Could you check a few things on this model? Use its own coordinates, in mm. A direction names the side the tool comes from. Give positions to 0.01 mm unless a question says otherwise; leave off trailing zeros. Loops run counter-clockwise (first coordinate to the right, second up) from the corner with the lowest first, then second, coordinate; pieces in that order, holes last. Notation, with made-up numbers: (29, 47) - (57, 47) arc R10 cw to (57, 57) - close; hole circle Ø8 at (-4, 60.25). An arc over 180 degrees is marked (long way). Write each question's results on one line, items separated by ' | '. Start each with the question number.
```python
from build123d import *

# Parameters (mm, degrees)
EXTRUDE_1_DEPTH     = 12
SKETCH_3_W          = 26
SKETCH_3_H          = 12
CUT_EXTRUDE_1_DEPTH = 2
SKETCH_4_R          = 1.5
CUT_EXTRUDE_2_DEPTH = 7


with BuildPart() as part:
    # 草图2 → 凸台-拉伸1 (new body)
    with BuildSketch(Plane(origin=(0, 0, 0), x_dir=(1, 0, 0), z_dir=(0, 1, 0))):
        Polygon((-13, 0), (-9.07179677, 0), (-8, 4), (8, 4), (9.07179677, 0), (13, 0), (13, 9), (-13, 9), align=None)
    extrude(amount=EXTRUDE_1_DEPTH)

    # 草图3 → 切除-拉伸1 (cut)
    with BuildSketch(Plane(origin=(0, 0, -9), x_dir=(-1, 0, 0), z_dir=(0, 0, -1))):
        with Locations((0, 6)):
            Rectangle(SKETCH_3_W, SKETCH_3_H)
    extrude(amount=-CUT_EXTRUDE_1_DEPTH, mode=Mode.SUBTRACT)

    # 草图4 → 切除-拉伸2 (cut)
    with BuildSketch(Plane(origin=(0, 0, -7), x_dir=(-1, 0, 0), z_dir=(0, 0, -1))):
        with Locations((-11, 3)):
            Circle(SKETCH_4_R)
        with Locations(Location((11, 3, 0), (0, 0, 180))):
            Circle(SKETCH_4_R)
        with Locations((11, 9)):
            Circle(SKETCH_4_R)
        with Locations(Location((-11, 9, 0), (0, 0, 180))):
            Circle(SKETCH_4_R)
    extrude(amount=-CUT_EXTRUDE_2_DEPTH, mode=Mode.SUBTRACT)


solid = part.part
```
Q1. If we mould it in two halves opening along X, with no side actions, what happens to faces 3 (the face through (-0.2, 12, -4.3)), 4 (the face through (0, 6, -4)), 5 (the face through (8.528, 5.916, -2.028)), 6 (the face through (-13, 6, -4))? For each: +X half, -X half, draft (parallel to the pull), parting line (faces both ways), or undercut.
Q2. I need wall thicknesses on L1, parallel to Y at x = -11, z = -1.75; L2, parallel to Z at x = 2.75, y = 8; L3, parallel to X at y = 11.5, z = -1.25. Which ranges of each line are inside material? Lowest first, please. Write a range as from..to.
Q3. I want a section at D-D, the plane z = -6.5. List the corners of the cut face in (x, y) for me.
Q4. I want a section at B-B, the plane z = -1. List the corners of the cut face in (x, y) for me.
Q5. Which directions (+Z, -Z, +X, -X, +Y, -Y) give clear straight access to the entire face, cutting with the end or side of a thin tool? Please do faces 1 (the face through (12.2, 2.1, -3.5)), 2 (the face through (-8.543, 5.916, -1.972)).
Q6. I want a section at A-A, the plane y = 3. List the corners of the cut face in (x, z) for me, then the cut area to 3 significant figures.
Q7. I want a section at C-C, the plane x = 11. List the corners of the cut face in (y, z) for me, then the cut area to 3 significant figures.
Conclusion:
1) face 3: draft | face 4: undercut | face 5: undercut | face 6: -X half
2) L1: 0..1.5, 4.5..7.5, 10.5..12 | L2: -7..-4 | L3: -13..-8.74, 8.74..13
3) outline: (-13, 0) - (13, 0) - (13, 12) - (-13, 12) - close; hole circle Ø3 at (-11, 3); hole circle Ø3 at (-11, 9); hole circle Ø3 at (11, 3); hole circle Ø3 at (11, 9)
4) outline: (-13, 0) - (-8.8, 0) - (-8.8, 12) - (-13, 12) - close; (8.8, 0) - (13, 0) - (13, 12) - (8.8, 12) - close; hole circle Ø3 at (-11, 3); hole circle Ø3 at (-11, 9); hole circle Ø3 at (11, 3); hole circle Ø3 at (11, 9)
5) face 1: +Z, -Z | face 2: +Z, +Y, -Y
6) outline: (-13, -7) - (-12.5, -7) - (-12.5, 0) - (-13, 0) - close; (-9.5, -7) - (9.5, -7) - (9.5, 0) - (9.07, 0) - (8, -4) - (-8, -4) - (-9.07, 0) - (-9.5, 0) - close; (12.5, -7) - (13, -7) - (13, 0) - (12.5, 0) - close | area: 71.7 mm^2
7) outline: (0, -7) - (1.5, -7) - (1.5, 0) - (0, 0) - close; (4.5, -7) - (7.5, -7) - (7.5, 0) - (4.5, 0) - close; (10.5, -7) - (12, -7) - (12, 0) - (10.5, 0) - close | area: 42.0 mm^2
